Here's how the part is built. I have some questions about the finished solid (model axes, mm). A direction names the side the tool comes from. Round coordinates to 2 decimals unless told otherwise and drop trailing zeros. Loops run counter-clockwise (first coordinate to the right, second up) from the corner with the lowest first, then second, coordinate; pieces in that order, holes last. Notation, with made-up numbers: M 53.5,70.25 L 66.5,70.25 A24 ccw 66.5,109.25 Z; hole C 79,-30 d2. An arc over 180 degrees is marked long. Answer as a JSON object with one key per item and string values.
from build123d import *

# Parameters (mm, degrees)
BOSS_EXTRUDE1_DEPTH = 8
SKETCH2_W           = 60
SKETCH2_H           = 3
CUT_EXTRUDE1_DEPTH  = 4
SKETCH3_R           = 4
SKETCH3_R_2         = 3
CUT_EXTRUDE3_DEPTH  = 5.5
BOSS_EXTRUDE3_START = 45
SKETCH4_R           = 4.5
SKETCH4_R_2         = 3
BOSS_EXTRUDE3_DEPTH = 45
SKETCH6_R           = 25
SKETCH6_R_2         = 24
BOSS_EXTRUDE4_DEPTH = 30


with BuildPart() as part:
    # Sketch1 → Boss-Extrude1 (new body)
    with BuildSketch(Plane.XY):
        with BuildLine():
            Line((-30, 30), (30, 30))
            ThreePointArc((30, 30), (60, 0), (30, -30))
            Line((30, -30), (-30, -30))
            ThreePointArc((-30, -30), (-60, 0), (-30, 30))
        make_face()
    extrude(amount=BOSS_EXTRUDE1_DEPTH)

    # Sketch2 → Cut-Extrude1 (cut, symmetric)
    with BuildSketch(Plane(origin=(0, 0, 0), x_dir=(1, 0, 0), z_dir=(0, 1, 0))):
        with Locations((0, -4)):
            Rectangle(SKETCH2_W, SKETCH2_H)
    extrude(amount=CUT_EXTRUDE1_DEPTH, both=True, mode=Mode.SUBTRACT)

    # Sketch3 → Cut-Extrude3 (cut)
    with BuildSketch(Plane.XY.offset(8)):
        with Locations((30, 0)):
            Circle(SKETCH3_R)
        with Locations((-30, 0)):
            Circle(SKETCH3_R_2)
    extrude(amount=-CUT_EXTRUDE3_DEPTH, mode=Mode.SUBTRACT)

    # Sketch4 → Boss-Extrude3 (add)
    with BuildSketch(Plane.XY.offset(8).offset(BOSS_EXTRUDE3_START)):
        with Locations(Location((-30, 0, 0), (0, 0, 180))):
            Circle(SKETCH4_R)
        with Locations((-30, 0)):
            Circle(SKETCH4_R_2, mode=Mode.SUBTRACT)
    extrude(amount=-BOSS_EXTRUDE3_DEPTH)

    # Sketch5 → Revolve1 (revolve)
    with BuildSketch(Plane(origin=(0, 0, 0), x_dir=(1, 0, 0), z_dir=(0, 1, 0)), mode=Mode.PRIVATE) as revolve1_sk:
        Polygon((-33, -52.999308425), (-33, -50.999308425), (-31, -52.499308425), (-31, -52.999308425), align=None)
    revolve(revolve1_sk.sketch.rotate(Axis((-30, 0, 53), (0, 0, 1)), 90), axis=Axis((-30, 0, 53), (0, 0, 1)))

    # Sketch6 → Boss-Extrude4 (add)
    with BuildSketch(Plane.XY.offset(8)):
        with Locations((30, 0)):
            Circle(SKETCH6_R)
        with Locations((30, 0)):
            Circle(SKETCH6_R_2, mode=Mode.SUBTRACT)
    extrude(amount=BOSS_EXTRUDE4_DEPTH)


solid = part.part
Item 1: I want a section at C-C, the plane y = 15.5. Please give me the cut outline in (x, z), then the cut area to 3 significant figures.
Resolved:
{"outline": "M -55.69,0 L 55.69,0 L 55.69,8 L 49.62,8 L 49.62,38 L 48.32,38 L 48.32,8 L 11.68,8 L 11.68,38 L 10.38,38 L 10.38,8 L -55.69,8 Z", "area": "968 mm²"}
Item 2: Please list where these lines run through material, in increasing order: probe 1 along X at (y, z) = (0, 4.25); probe 2 along Y at (x, z) = (-30, 40); probe 3 along Z at (x, y) = (-44.5, -11). Write a range as from..to.
Resolved:
{"probe 1": "-60..-33, 34..60", "probe 2": "-4.5..-3, 3..4.5", "probe 3": "0..8"}
Item 3: I want a section at D-D, the plane z = 49.5. Please give me the cut outline in (x, y), then the cut area to 3 significant figures.
Resolved:
{"outline": "C -30,0 d9; hole C -30,0 d6", "area": "35.3 mm²"}
Item 4: I want a section at A-A, the plane x = -5. Please give me the cut outline in (y, z).
Resolved:
{"outline": "M -30,0 L 30,0 L 30,8 L -30,8 Z; hole M -4,2.5 L 4,2.5 L 4,5.5 L -4,5.5 Z"}
Item 5: I'm going to push flat-ended pins straight in: pin 1 Ø6 at (x, z) = (-30, 16.5) entering from -Y; pin 2 Ø1 at (x, y) = (32, -10) entering from +Z; pin 3 Ø9 at (x, y) = (-11.5, -1) entering from -Z; pin 4 Ø6 at (y, z) = (8, 28) entering from +X. Where does each tip first touch, or does it pass through?
Resolved:
{"pin 1": "y = -4.5", "pin 2": "z = 8", "pin 3": "z = 0", "pin 4": "x = 54.49"}
Item 6: If we mould it in two halves opening along Y, with no side actions, what happens to faces 1 (the face through (-12, 0, 8)), 2 (the face through (0, -30, 4)), 3 (the face through (0, 4, 4)), 4 (the face through (0, 0, 5.5))? For each: pulls with the +Y half, pulls with the -Y half, needs draft (parallel to the pull), parting line crosses it, or undercut.
Resolved:
{"face 1": "needs draft", "face 2": "pulls with the -Y half", "face 3": "undercut", "face 4": "undercut"}
Item 7: On a 3-axis mill with a long thin cutter (end or side, diameter ignored), from which of +Z, -Z, +X, -X, +Y, -Y can I reach the whole of each face in a straight line? I mean faces 5 (the face through (-59.993, -0.66, 3.944)), 6 (the face through (0, -4, 4)), 7 (the face through (11.574, 16.896, 22.79)), 8 (the face through (7.7, 9.4, 38)). Say none if no direction works.
Resolved:
{"face 5": "+Z, -Z, -X", "face 6": "none", "face 7": "+Z", "face 8": "+Z, +X, +Y, -Y"}
Item 8: I want a section at B-B, the plane z = 27.5. Please give me the cut outline in (x, y), then the cut area to 3 significant figures.
Resolved:
{"outline": "C -30,0 d9; C 30,0 d50; hole C -30,0 d6; hole C 30,0 d48", "area": "189 mm²"}
